Autodesk Inventor part; units mm, degrees
ref_plane "YZ Plane" through (0, 0, 0) normal (1, 0, 0) x (0, 1, 0)
ref_plane "XZ Plane" through (0, 0, 0) normal (0, 1, 0) x (-1, 0, 0)
ref_plane "XY Plane" through (0, 0, 0) normal (0, 0, 1) x (1, 0, 0)
sketch "Sketch1" plane through (0, 0, 0) normal (0, 0, 1) x (1, 0, 0)
  circle A0 centre (0, 0) radius 25 construction
  line L0 (0, 0) -> (0, 25) construction
  line L1 (0, 0) -> (21.6506, -12.5) construction
  line L2 (0, 0) -> (-21.6506, -12.5) construction
  line L3 (0, 25) -> (8, 25)
  line L4 (0, 25) -> (-8, 25)
  line L5 (0, 25) -> (8, 25) construction
  line L6 (21.6506, -12.5) -> (25.6506, -5.5718)
  line L7 (21.6506, -12.5) -> (29.6506, -12.5) construction
  line L8 (21.6506, -12.5) -> (17.6506, -19.4282)
  line L9 (21.6506, -12.5) -> (29.6506, -12.5) construction
  line L10 (-21.6506, -12.5) -> (-25.6506, -5.5718)
  line L11 (-21.6506, -12.5) -> (-13.6506, -12.5) construction
  line L12 (-21.6506, -12.5) -> (-17.6506, -19.4282)
  line L13 (-21.6506, -12.5) -> (-13.6506, -12.5) construction
  line L14 (8, 25) -> (8, 34.0735)
  line L15 (-8, 25) -> (-8, 34.0735)
  line L16 (25.6506, -5.5718) -> (33.5085, -10.1085)
  line L17 (17.6506, -19.4282) -> (25.5085, -23.9649)
  line L18 (-17.6506, -19.4282) -> (-25.5085, -23.9649)
  line L19 (-25.6506, -5.5718) -> (-33.5085, -10.1085)
  arc A1 (33.5085, -10.1085) -> (8, 34.0735) centre (0, 0) ccw
  arc A2 (-8, 34.0735) -> (-33.5085, -10.1085) centre (0, 0) ccw
  arc A3 (-25.5085, -23.9649) -> (25.5085, -23.9649) centre (0, 0) ccw
  dimension "d0" = 50
  dimension "d1" = 120
  dimension "d2" = 120
  dimension "d3" = 8
  dimension "d4" = 8
  dimension "d5" = 180
  dimension "d6" = 8
  dimension "d7" = 60
  dimension "d8" = 8
  dimension "d9" = 120
  dimension "d10" = 8
  dimension "d11" = 120
  dimension "d12" = 8
  dimension "d13" = 60
  dimension "d15" = 35
  dimension "d16" = 35
  dimension "d17" = 35
extrude "Extrusion1" add sketch "Sketch1" along normal blind 21
sketch "Sketch2" plane through (0, 0, 21) normal (0, 0, 1) x (1, 0, 0)
  line L0 (-17.5, -17.5) -> (17.5, -17.5)
  line L1 (17.5, -17.5) -> (17.5, 17.5)
  line L2 (17.5, 17.5) -> (-17.5, 17.5)
  line L3 (-17.5, 17.5) -> (-17.5, -17.5)
  line L4 (-17.5, -17.5) -> (17.5, 17.5) construction
  line L5 (17.5, -17.5) -> (-17.5, 17.5) construction
  point P0 (0, 0)
  dimension "d20" = 35
  dimension "d21" = 35
extrude "Extrusion2" add sketch "Sketch2" along normal blind 79
fillet "Fillet1" radius 5 4 edges at (17.5, 17.5, 60.5) (17.5, -17.5, 60.5) (-17.5, 17.5, 60.5) (-17.5, -17.5, 60.5)
fillet "Fillet2" radius 1 37 edges at (30.3109, 17.5, 0) (-30.3109, 17.5, 0) (0, -35, 0) (21.6506, -12.5, 0) (29.5796, -7.8402, 0) (21.5796, -21.6966, 0) (8, 29.5367, 0) (0, 25, 0) (-8, 29.5367, 0) (-29.5796, -7.8402, 0) (-21.6506, -12.5, 0) (-21.5796, -21.6966, 0) (16.0355, 16.0355, 21) (17.5, 0, 21) (16.0355, -16.0355, 21) (0, -17.5, 21) (-16.0355, -16.0355, 21) (-17.5, 0, 21) (-16.0355, 16.0355, 21) (0, 17.5, 21) (0, 25, 21) (8, 29.5367, 21) (30.3109, 17.5, 21) (8, 34.0735, 10.5) (-8, 34.0735, 10.5) (-30.3109, 17.5, 21) (21.6506, -12.5, 21) (29.5796, -7.8402, 21) (33.5085, -10.1085, 10.5) (21.5796, -21.6966, 21) (25.5085, -23.9649, 10.5) (0, -35, 21) (-21.5796, -21.6966, 21) (-21.6506, -12.5, 21) (-29.5796, -7.8402, 21) (-33.5085, -10.1085, 10.5) (-25.5085, -23.9649, 10.5)
sketch "Sketch4" plane through (0, 0, 100) normal (0, 0, 1) x (1, 0, 0)
  line L0 (-100, 9) -> (100, 9)
  line L1 (100, 9) -> (100, -9)
  line L2 (100, -9) -> (-100, -9)
  line L3 (-100, -9) -> (-100, 9)
  line L4 (-100, 9) -> (100, -9) construction
  line L5 (100, 9) -> (-100, -9) construction
  point P0 (0, 0)
  dimension "d29" = 200
  dimension "d30" = 18
extrude "Extrusion4" add sketch "Sketch4" along normal blind 20
chamfer "Chamfer1" distance 15 distance2 7.5 1 edges at (0, 9, 120) measured on face at (-5.8333, 9, 113.3333)
chamfer "Chamfer2" distance 15 distance2 7.5 1 edges at (0, -9, 120) measured on face at (5.8333, -9, 113.3333)
sketch "Sketch5" plane through (-17.5, -12.5, 22) normal (-1, 0, 0) x (0, 0, 1)
  line L0 (78, 25) -> (78, 21.5)
  line L1 (78, 21.5) -> (59, 30)
  line L2 (78, 30) -> (0, 30)
  line L3 (78, 21.5) -> (78, 3.5)
  line L4 (78, 3.5) -> (59, -5)
  line L5 (0, -5) -> (78, -5)
  line L6 (-1, 45.5377) -> (-1, 3.9006)
  line L7 (-1, -11.6878) -> (-1, -21.5)
  line L8 (59, 30) -> (79.7538, 33.0683)
  line L9 (79.7538, 33.0683) -> (78, 21.5)
  line L10 (78, 0) -> (78, 3.5)
  line L11 (78, 3.5) -> (84.2924, -8.3159)
  line L12 (84.2924, -8.3159) -> (59, -5)
  point P0 (-22, 12.5)
  dimension "d39" = 60
  dimension "d40" = 60
extrude "Extrusion5" cut sketch "Sketch5" against normal through all
equation "\"d3\" = d4"
equation "\"d6\" = d4"
equation "\"d8\" = d4"
equation "\"d10\" = d4"
equation "\"d12\" = d4"
equation "\"d16\" = d15"
equation "\"d17\" = d15"
equation "\"d40\" = d39"
properties part number "Squeegee"
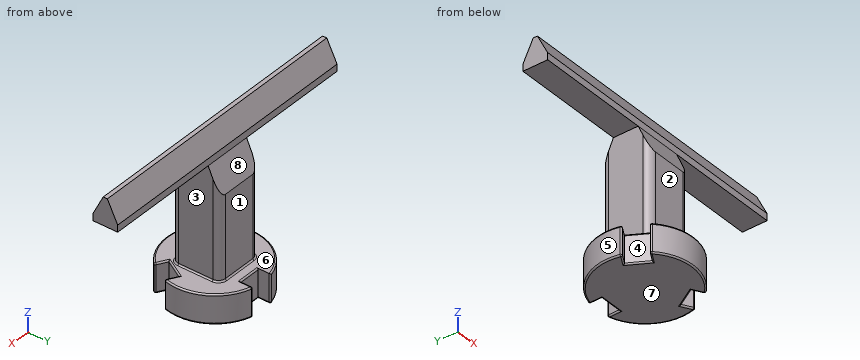
The model under review builds one solid part; all positions refer to its coordinate system, in mm. Face numbers are marked on the shaded views. A direction names the side the tool comes from. Round coordinates to 2 decimals unless told otherwise and drop trailing zeros. Loops run counter-clockwise (first coordinate to the right, second up) from the corner with the lowest first, then second, coordinate; pieces in that order, holes last. Notation, with made-up numbers: M -29.75,6 L 1.25,6 A7 cw 1.25,10 Z; hole C 36.5,40 d7. An arc over 180 degrees is marked long. Answer as CSV lines item,"result". Start each with the question number.
Item 1: Consider section D-D (z = 89). Write out the cut boundary in (x, y).
Item 2: Consider section A-A (z = 46). Write out the cut boundary in (x, y).
Item 3: Wall thickness on line 1 (X direction, y = -1.5, z = 36); line 2 (Z direction, x = -5.5, y = -19); line 3 (Z direction, x = -67, y = -1.5): over which ranges is each line inside the solid? List them lowest first. Write a range as [from, to].
Item 4: Insertion check: P1, Ø7.5, axis at y = -4.5, z = 51.5, coming from the +X side; P2, Ø4, axis at x = -35, z = 101.5, coming from the -Y side; P3, Ø12.5, axis at y = 5, z = 46, coming from the -X side. Each pin has a flat end and moves straight along its axis. Give the tip position at first contact, or say it passes through.
Item 5: For the marked faces 1, 2, 3 and 4, list the 3-axis set-ups (+Z, -Z, +X, -X, +Y, -Y) from which the entire face can be reached by the end or side of a thin tool; tool diameter is ignored.
Item 6: Consider section C-C (z = 15). Write out the cut boundary in (x, y), then the cut area to 3 significant figures.
Item 7: Mouldability with a two-part tool opening along Z and no side actions: class the marked faces 5, 6, 7 and 8 as released by +Z, released by -Z, zero draft, split by the parting line, or undercut.
Item 8: Consider section B-B (x = 74.5). Write out the cut boundary in (y, z).
Answer:
1,outline,"M -17.5,-12.5 A5 ccw -17.29,-13.92 L 17.29,-13.92 A5 ccw 17.5,-12.5 L 17.5,12.5 A5 ccw 17.29,13.92 L -17.29,13.92 A5 ccw -17.5,12.5 Z"
2,outline,"M -17.5,-12.5 A5 ccw -12.5,-17.5 L 12.5,-17.5 A5 ccw 17.5,-12.5 L 17.5,12.5 A5 ccw 12.5,17.5 L -12.5,17.5 A5 ccw -17.5,12.5 Z"
3,line 1,"x = [-17.5, 17.5]"
3,line 2,"z = [0, 21]"
3,line 3,"z = [100, 120]"
4,P1,"stops at x = 17.5"
4,P2,"stops at y = -9"
4,P3,"stops at x = -17.5"
5,face 1,"+Z, +X, -X, +Y"
5,face 2,"+Z, +X, -X, -Y"
5,face 3,"+X, +Y, -Y"
5,face 4,"-Z"
6,outline,"M -33.86,-8.85 A1 ccw -32.39,-9.47 L -25.65,-5.57 L -17.65,-19.43 L -24.39,-23.32 A1 ccw -24.6,-24.9 A35 ccw 24.6,-24.9 A1 ccw 24.39,-23.32 L 17.65,-19.43 L 25.65,-5.57 L 32.39,-9.47 A1 ccw 33.86,-8.85 A35 ccw 9.26,33.75 A1 ccw 8,32.79 L 8,25 L -8,25 L -8,32.79 A1 ccw -9.26,33.75 A35 ccw Z"
6,area,"3,380 mm^2"
7,face 5,"zero draft"
7,face 6,"undercut"
7,face 7,"released by -Z"
7,face 8,"released by +Z"
8,outline,"M -9,100 L 9,100 L 9,105 L 1.5,120 L -1.5,120 L -9,105 Z"
